Geometry: final body of the model. Coordinates: model frame, mm. Coordinates: 2 decimals unless noted, no trailing zeros. Loops run counter-clockwise (first coordinate to the right, second up) from the corner with the lowest first, then second, coordinate; pieces in that order, holes last. Notation, with made-up numbers: (-15, -6.5) - (-2, -6.5) arc R21 cw to (-2, 11.5) - close; hole circle Ø8 at (44, -27). An arc over 180 degrees is marked (long way). Answer in a Markdown table with one row per item.
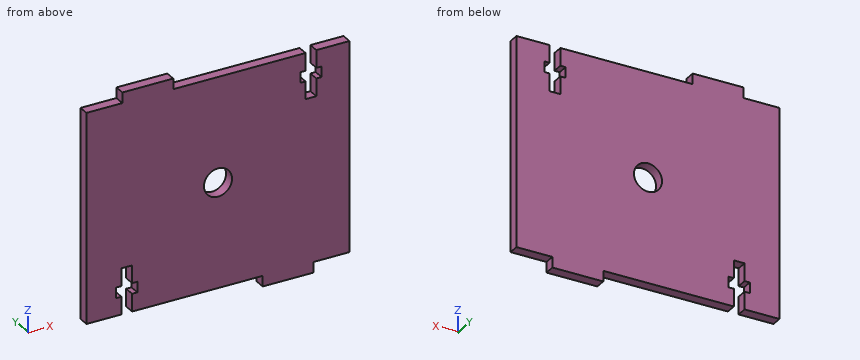
from build123d import *

# Parameters (mm, degrees)
ESQUISSE3_W        = 14.5
ESQUISSE3_H        = 3
ESQUISSE3_R        = 4
BOSS_EXTRU_1_DEPTH = 3


with BuildPart() as part:
    # Esquisse3 → Boss.-Extru.1 (new body)
    # profile 1 of 3: a face of its own
    with BuildSketch(Plane(origin=(0, 0, 0), x_dir=(1, 0, 0), z_dir=(0, 1, 0))):
        with Locations((17.5, -1.5)):
            Rectangle(ESQUISSE3_W, ESQUISSE3_H)
    # profile 2 of 3: a face of its own
    with BuildSketch(Plane(origin=(0, 0, 0), x_dir=(1, 0, 0), z_dir=(0, 1, 0))):
        Polygon((0, 59.5), (0, 0), (10.25, 0), (24.75, 0), (62.484051244, 0), (62.484051244, 5), (60.984051244, 5), (60.984051244, 8), (62.484051244, 8), (62.484051244, 13), (65.541555924, 13), (65.541555924, 8), (67.041555924, 8), (67.041555924, 5), (65.541555924, 5), (65.541555924, 0), (75, 0), (75, 59.5), (64.75, 59.5), (50.25, 59.5), (13.015948756, 59.5), (13.015948756, 54.5), (14.515948756, 54.5), (14.515948756, 51.5), (13.015948756, 51.5), (13.015948756, 46.5), (9.958444076, 46.5), (9.958444076, 51.5), (8.458444076, 51.5), (8.458444076, 54.5), (9.958444076, 54.5), (9.958444076, 59.5), align=None)
        with Locations(Location((37.5, 29.75, 0), (0, 0, 270))):
            Circle(ESQUISSE3_R, mode=Mode.SUBTRACT)
    # profile 3 of 3: a face of its own
    with BuildSketch(Plane(origin=(0, 0, 0), x_dir=(1, 0, 0), z_dir=(0, 1, 0))):
        with Locations((57.5, 61)):
            Rectangle(ESQUISSE3_W, ESQUISSE3_H)
    extrude(amount=BOSS_EXTRU_1_DEPTH)


solid = part.part
(1) First-contact query: pin 1 Ø0.8 at (x, y) = (61.5, 2) entering from +Z; pin 2 Ø1.5 at (x, y) = (64.5, 2) entering from +Z; pin 3 Ø0.9 at (y, z) = (1.5, -61.5) entering from -X. Flat tips, straight axial feed; report the tip coordinate or a pass-through.
Verdict:
| item | result |
|---|---|
| pin 1 | stops at z = 0 |
| pin 2 | stops at z = -13 |
| pin 3 | stops at x = 50.25 |
(2) Cut plane B-B on z = -29.75. Output: boundary loops of the cut face in (x, y).
Verdict:
| item | result |
|---|---|
| outline | (0, 0) - (33.5, 0) - (33.5, 3) - (0, 3) - close; (41.5, 0) - (75, 0) - (75, 3) - (41.5, 3) - close |
(3) Ray query, probe 1 along X at (y, z) = (1.2, -29.75); probe 2 along X at (y, z) = (2.6, -6.5); probe 3 along Z at (x, y) = (50, 1.5). Return the intervals inside material, ascending.
Verdict:
| item | result |
|---|---|
| probe 1 | x = 0 to 33.5, 41.5 to 75 |
| probe 2 | x = 0 to 60.98, 67.04 to 75 |
| probe 3 | z = -59.5 to 0 |
(4) Cut plane C-C on x = 23.5. Output: boundary loops of the cut face in (y, z).
Verdict:
| item | result |
|---|---|
| outline | (0, -59.5) - (3, -59.5) - (3, 3) - (0, 3) - close |
(5) Cut plane D-D on x = 12. Output: boundary loops of the cut face in (y, z), then the cut area to 4 significant figures.
Verdict:
| item | result |
|---|---|
| outline | (0, -46.5) - (3, -46.5) - (3, 3) - (0, 3) - close |
| area | 148.5 mm² |
(6) Cut plane A-A on x = 37.5. Output: boundary loops of the cut face in (y, z), then the cut area to 4 significant figures.
Verdict:
| item | result |
|---|---|
| outline | (0, -59.5) - (3, -59.5) - (3, -33.75) - (0, -33.75) - close; (0, -25.75) - (3, -25.75) - (3, 0) - (0, 0) - close |
| area | 154.5 mm² |
